Job drawing, mm, ordinate dimensions from the low corner. One solid piece. Coordinates: 2 decimals unless noted, no trailing zeros. Order: outer loops, then holes, each group sorted by start corner. A loop starts at its lowest first (then second) coordinate and runs counter-clockwise, first axis right, second up. Notation, with made-up numbers: (44, 34) - (80, 34) arc R23 ccw to (80, 57) - close; hole circle Ø8 at (9, -36.5). An arc over 180 degrees is marked (long way). Use a Markdown table: item, result. Add a question column.
1) Saw through at A-A on y = 2.25. List the corners of the cut face in (x, z).
2) Saw through at C-C on x = 77.5. List the corners of the cut face in (y, z).
3) Saw through at B-B on z = 85. List the corners of the cut face in (x, y).
4) Drop flat-ended pins along their axis: P1, Ø8, axis at y = 22, z = 113, coming from the -X side; P2, Ø3, axis at x = 76.5, y = 19, coming from the +Z side; P3, Ø1, axis at y = 13, z = 27.5, coming from the -X side. Give the stop position or say it passes through.
5) Saw through at D-D on x = 20. List the corners of the cut face in (y, z).
6) Two-plate mould, pull along X, no slides. Class the marked faces 1, 2 and 3: +X half, -X half, draft (parallel to the pull), parting line (faces both ways), or undercut.
7) Wall check: L1, parallel to Z at x = 77.5, y = 6.5; L2, parallel to X at y = 4.5, z = 84. Give the ranges that are in metal, low to high. Write a range as [from, to].
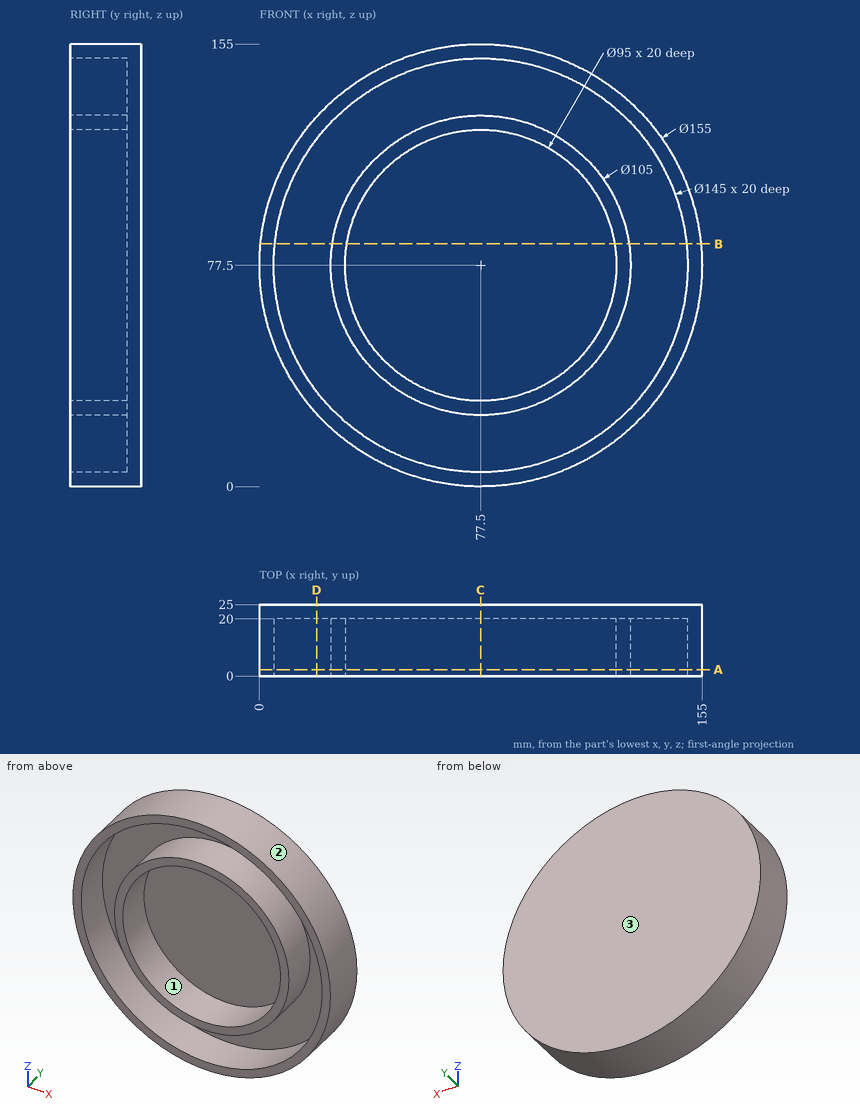
Results are:
| question | item | result |
|---|---|---|
| 1 | outline | circle Ø155 at (77.5, 77.5); circle Ø105 at (77.5, 77.5); hole circle Ø145 at (77.5, 77.5); hole circle Ø95 at (77.5, 77.5) |
| 2 | outline | (0, 0) - (25, 0) - (25, 155) - (0, 155) - (0, 150) - (20, 150) - (20, 130) - (0, 130) - (0, 125) - (20, 125) - (20, 30) - (0, 30) - (0, 25) - (20, 25) - (20, 5) - (0, 5) - close |
| 3 | outline | (0.36, 0) - (5.39, 0) - (5.39, 20) - (25.54, 20) - (25.54, 0) - (30.6, 0) - (30.6, 20) - (124.4, 20) - (124.4, 0) - (129.46, 0) - (129.46, 20) - (149.61, 20) - (149.61, 0) - (154.64, 0) - (154.64, 25) - (0.36, 25) - close |
| 4 | P1 | x = 6.69 |
| 4 | P2 | z = 155 |
| 4 | P3 | x = 17.87 |
| 5 | outline | (0, 25.54) - (25, 25.54) - (25, 129.46) - (0, 129.46) - (0, 121.66) - (20, 121.66) - (20, 33.34) - (0, 33.34) - close |
| 6 | face 1 | undercut |
| 6 | face 2 | parting line |
| 6 | face 3 | draft |
| 7 | L1 | [0, 5], [25, 30], [125, 130], [150, 155] |
| 7 | L2 | [0.27, 5.29], [25.4, 30.45], [124.55, 129.6], [149.71, 154.73] |
